from build123d import *

# Parameters (mm, degrees)
SKETCH1_W           = 76
SKETCH1_H           = 76
BOSS_EXTRUDE1_DEPTH = 110
SKETCH2_W           = 60
SKETCH2_H           = 60
CUT_EXTRUDE1_DEPTH  = 100
CUT_EXTRUDE2_REACH  = 140.996
CUT_EXTRUDE3_REACH  = 140.996


with BuildPart() as part:
    # Sketch1 → Boss-Extrude1 (new body)
    with BuildSketch(Plane.XY):
        Rectangle(SKETCH1_W, SKETCH1_H)
    extrude(amount=BOSS_EXTRUDE1_DEPTH)

    # Sketch2 → Cut-Extrude1 (cut)
    with BuildSketch(Plane.XY.offset(110)):
        Rectangle(SKETCH2_W, SKETCH2_H)
    extrude(amount=-CUT_EXTRUDE1_DEPTH, mode=Mode.SUBTRACT)

    # Cut-Extrude2: up to this face of the body (flat: up to its plane)
    cut_extrude2_end = Plane(part.part.faces().sort_by_distance((0, -38, 55))[0])
    # Sketch4 → Cut-Extrude2 (cut, up to the picked face)
    with BuildSketch(Plane(origin=(0, 38, 0), x_dir=(1, 0, 0), z_dir=(0, 1, 0)), mode=Mode.PRIVATE) as cut_extrude2_sk1:
        Polygon((-26.229048752, -10), (0, -47.963096879), (26.229048752, -10), align=None)
    cut_extrude2_tool1 = split(extrude(cut_extrude2_sk1.sketch, amount=-CUT_EXTRUDE2_REACH, mode=Mode.PRIVATE), bisect_by=cut_extrude2_end, keep=Keep.BOTH, mode=Mode.PRIVATE)
    # Sketch4 → Cut-Extrude2 (cut, up to the picked face)
    with BuildSketch(Plane(origin=(0, 38, 0), x_dir=(1, 0, 0), z_dir=(0, 1, 0)), mode=Mode.PRIVATE) as cut_extrude2_sk2:
        Polygon((0, -62.036903121), (26.229048752, -100), (-26.229048752, -100), align=None)
    cut_extrude2_tool2 = split(extrude(cut_extrude2_sk2.sketch, amount=-CUT_EXTRUDE2_REACH, mode=Mode.PRIVATE), bisect_by=cut_extrude2_end, keep=Keep.BOTH, mode=Mode.PRIVATE)
    # Sketch4 → Cut-Extrude2 (cut, up to the picked face)
    with BuildSketch(Plane(origin=(0, 38, 0), x_dir=(1, 0, 0), z_dir=(0, 1, 0)), mode=Mode.PRIVATE) as cut_extrude2_sk3:
        Polygon((4.861860338, -55), (30, -18.61585049), (30, -91.38414951), align=None)
    cut_extrude2_tool3 = split(extrude(cut_extrude2_sk3.sketch, amount=-CUT_EXTRUDE2_REACH, mode=Mode.PRIVATE), bisect_by=cut_extrude2_end, keep=Keep.BOTH, mode=Mode.PRIVATE)
    # Sketch4 → Cut-Extrude2 (cut, up to the picked face)
    with BuildSketch(Plane(origin=(0, 38, 0), x_dir=(1, 0, 0), z_dir=(0, 1, 0)), mode=Mode.PRIVATE) as cut_extrude2_sk4:
        Polygon((-30, -91.38414951), (-4.861860338, -55), (-30, -18.61585049), align=None)
    cut_extrude2_tool4 = split(extrude(cut_extrude2_sk4.sketch, amount=-CUT_EXTRUDE2_REACH, mode=Mode.PRIVATE), bisect_by=cut_extrude2_end, keep=Keep.BOTH, mode=Mode.PRIVATE)
    add(cut_extrude2_tool1.solids().sort_by(Axis((0, 38, 22.654366), (0, -1, 0)))[0], mode=Mode.SUBTRACT)
    add(cut_extrude2_tool2.solids().sort_by(Axis((0, 38, 87.345634), (0, -1, 0)))[0], mode=Mode.SUBTRACT)
    add(cut_extrude2_tool3.solids().sort_by(Axis((21.62062, 38, 55), (0, -1, 0)))[0], mode=Mode.SUBTRACT)
    add(cut_extrude2_tool4.solids().sort_by(Axis((-21.62062, 38, 55), (0, -1, 0)))[0], mode=Mode.SUBTRACT)

    # Cut-Extrude3: up to this face of the body (flat: up to its plane)
    cut_extrude3_end = Plane(part.part.faces().sort_by_distance((38, 0, 55))[0])
    # Sketch5 → Cut-Extrude3 (cut, up to the picked face)
    with BuildSketch(Plane.ZY.offset(38), mode=Mode.PRIVATE) as cut_extrude3_sk1:
        Polygon((18.61585049, 30), (55, 4.861860338), (91.38414951, 30), align=None)
    cut_extrude3_tool1 = split(extrude(cut_extrude3_sk1.sketch, amount=-CUT_EXTRUDE3_REACH, mode=Mode.PRIVATE), bisect_by=cut_extrude3_end, keep=Keep.BOTH, mode=Mode.PRIVATE)
    # Sketch5 → Cut-Extrude3 (cut, up to the picked face)
    with BuildSketch(Plane.ZY.offset(38), mode=Mode.PRIVATE) as cut_extrude3_sk2:
        Polygon((91.38414951, -30), (18.61585049, -30), (55, -4.861860338), align=None)
    cut_extrude3_tool2 = split(extrude(cut_extrude3_sk2.sketch, amount=-CUT_EXTRUDE3_REACH, mode=Mode.PRIVATE), bisect_by=cut_extrude3_end, keep=Keep.BOTH, mode=Mode.PRIVATE)
    # Sketch5 → Cut-Extrude3 (cut, up to the picked face)
    with BuildSketch(Plane.ZY.offset(38), mode=Mode.PRIVATE) as cut_extrude3_sk3:
        Polygon((10, 26.229048752), (47.963096879, 0), (10, -26.229048752), align=None)
    cut_extrude3_tool3 = split(extrude(cut_extrude3_sk3.sketch, amount=-CUT_EXTRUDE3_REACH, mode=Mode.PRIVATE), bisect_by=cut_extrude3_end, keep=Keep.BOTH, mode=Mode.PRIVATE)
    # Sketch5 → Cut-Extrude3 (cut, up to the picked face)
    with BuildSketch(Plane.ZY.offset(38), mode=Mode.PRIVATE) as cut_extrude3_sk4:
        Polygon((62.036903121, 0), (100, -26.229048752), (100, 26.229048752), align=None)
    cut_extrude3_tool4 = split(extrude(cut_extrude3_sk4.sketch, amount=-CUT_EXTRUDE3_REACH, mode=Mode.PRIVATE), bisect_by=cut_extrude3_end, keep=Keep.BOTH, mode=Mode.PRIVATE)
    add(cut_extrude3_tool1.solids().sort_by(Axis((-38, 21.62062, 55), (1, 0, 0)))[0], mode=Mode.SUBTRACT)
    add(cut_extrude3_tool2.solids().sort_by(Axis((-38, -21.62062, 55), (1, 0, 0)))[0], mode=Mode.SUBTRACT)
    add(cut_extrude3_tool3.solids().sort_by(Axis((-38, 0, 22.654366), (1, 0, 0)))[0], mode=Mode.SUBTRACT)
    add(cut_extrude3_tool4.solids().sort_by(Axis((-38, 0, 87.345634), (1, 0, 0)))[0], mode=Mode.SUBTRACT)


solid = part.part
CAD build for the part. Positions are in the model's coordinates, mm. A direction names the side the tool comes from. Coordinates: 2 decimals unless noted, no trailing zeros. Loops run counter-clockwise (first coordinate to the right, second up) from the corner with the lowest first, then second, coordinate; pieces in that order, holes last. Notation, with made-up numbers: (50, 44) - (75, 44) arc R5 cw to (75, 52) - close; hole circle Ø10 at (18, 81). An arc over 180 degrees is marked (long way). Write item = value, one per line. Start each with the question number.
Q1. Cut at C-C, the plane x = -22.5. List the corners of the cut face in (y, z), then the cut area to 3 significant figures.
Q2. Cut at B-B, the plane y = 2.5. List the corners of the cut face in (x, z).
Q3. Flat gauge pin, fed straight in: pin 1 Ø12 at (x, y) = (-22, 11) entering from +Z. Where does the tip first touch, or does it go through?
Q4. Which spindle directions (+Z, -Z, +X, -X, +Y, -Y) get a long thin tool onto all of the face, cutting with end or side? Do faces 4 (the flat face through (-34.056, 13.298, 28.716)), 5 (the flat face through (-13.298, -33.944, 28.716)), 6 (the flat face through (33, 1, 110)). Say none if no direction does.
Q5. Cut at D-D, the plane y = 23.5. List the corners of the cut face in (x, z).
Q6. Drill centre lines: L1, parallel to X at y = -20, z = 29; L2, parallel to Z at x = -5.5, y = 21.5. Where is each one in solid material? Low to high.
Q7. Pull direction Y, two halves, no side cores. Call faces 1 (the flat face through (-34.06, -17.61, 36.55)), 2 (the flat face through (-30, 34, 54)), 3 (the flat face through (-1, 38, 54)): pulls with the +Y half, pulls with the -Y half, needs draft (parallel to the pull), parting line crosses it, or undercut.
Q8. Cut at A-A, the plane z = 17. List the corners of the cut face in (x, y), then the cut area to 3 significant figures.
Computed:
q1.outline = (-38, 0) - (38, 0) - (38, 10) - (-38, 10) - close; (-38, 15.4) - (-30, 15.4) - (-30, 29.47) - (-38, 29.47) - close; (-38, 80.53) - (-30, 80.53) - (-30, 94.6) - (-38, 94.6) - close; (-38, 100) - (-30, 100) - (-30, 110) - (-38, 110) - close; (30, 15.4) - (38, 15.4) - (38, 29.47) - (30, 29.47) - close; (30, 80.53) - (38, 80.53) - (38, 94.6) - (30, 94.6) - close; (30, 100) - (38, 100) - (38, 110) - (30, 110) - close
q1.area = 1,370 mm²
q2.outline = (-38, 0) - (38, 0) - (38, 10) - (-38, 10) - close; (-38, 44.34) - (-30, 44.34) - (-30, 65.66) - (-38, 65.66) - close; (-38, 100) - (-30, 100) - (-30, 110) - (-38, 110) - close; (30, 44.34) - (38, 44.34) - (38, 65.66) - (30, 65.66) - close; (30, 100) - (38, 100) - (38, 110) - (30, 110) - close
q3.pin_1 = 10
q4.face_4 = +X, -X
q4.face_5 = +Y, -Y
q4.face_6 = +Z, +X, -X, +Y, -Y
q5.outline = (-38, 0) - (38, 0) - (38, 10) - (-38, 10) - close; (-38, 13.95) - (-30, 13.95) - (-30, 28.02) - (-38, 28.02) - close; (-38, 81.98) - (-30, 81.98) - (-30, 96.05) - (-38, 96.05) - close; (-38, 100) - (-30, 100) - (-30, 110) - (-38, 110) - close; (30, 13.95) - (38, 13.95) - (38, 28.02) - (30, 28.02) - close; (30, 81.98) - (38, 81.98) - (38, 96.05) - (30, 96.05) - close; (30, 100) - (38, 100) - (38, 110) - (30, 110) - close
q6.L1 = -38 to -30, 30 to 38
q6.L2 = 0 to 10
q7.face_1 = undercut
q7.face_2 = needs draft
q7.face_3 = pulls with the +Y half
q8.outline = (-38, -38) - (-21.39, -38) - (-21.39, -30) - (-30, -30) - (-30, -21.39) - (-38, -21.39) - close; (-38, 21.39) - (-30, 21.39) - (-30, 30) - (-21.39, 30) - (-21.39, 38) - (-38, 38) - close; (21.39, -38) - (38, -38) - (38, -21.39) - (30, -21.39) - (30, -30) - (21.39, -30) - close; (21.39, 30) - (30, 30) - (30, 21.39) - (38, 21.39) - (38, 38) - (21.39, 38) - close
q8.area = 807 mm²
